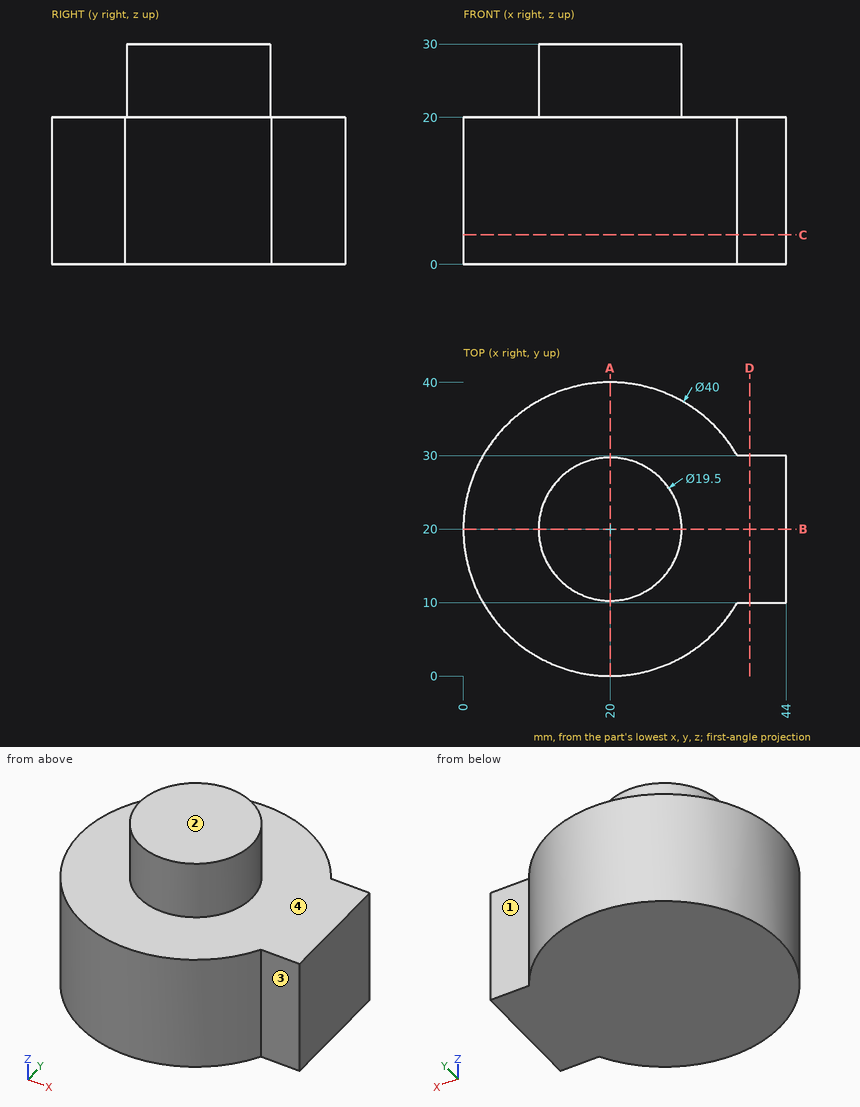
Check sheet for the drawn part. Datum: minimum x, y, z corner. Units: mm. A direction names the side the tool comes from. Coordinates: 2 decimals unless noted, no trailing zeros. Order: outer loops, then holes, each group sorted by start corner. A loop starts at its lowest first (then second) coordinate and runs counter-clockwise, first axis right, second up. Notation, with made-up numbers: M 40,30.5 L 88,30.5 A29 cw 88,55.5 Z; hole C -28.75,17 d8. An arc over 180 degrees is marked long. One line per question, with ' | ' between items. Start each with the question number.
Item 1: Cross-section at C-C on z = 4. Enter the section's corners in (x, y), then the cut area to 3 significant figures.
Item 2: Cross-section at D-D on x = 39. Enter the section's corners in (y, z), then the cut area to 3 significant figures.
Item 3: Cross-section at B-B on y = 20. Enter the section's corners in (x, z), then the cut area to 4 significant figures.
Item 4: Gauge pin test, flat ends, axial feed: pin 1 (10 mm diameter, centred on y = 6.5, z = 17, fed in from -X); pin 2 (4 mm diameter, centred on x = 26.5, y = 6, fed in from +Z); pin 3 (2 mm diameter, centred on x = 4.5, z = 17, fed in from +Y) (3 decimals). Record the tip position at first contact, or that the pin passes through.
Item 5: Material ranges on L1, parallel to X at y = 20.5, z = 27; L2, parallel to X at y = 20, z = 1.5; L3, parallel to Z at x = 32, y = 22.5, recorded low to high. Write a range as [from, to].
Item 6: Set-up check for the marked faces 1, 2, 3 and 4: record each of +Z, -Z, +X, -X, +Y, -Y from which the full face is reachable in a straight line by a thin tool's end or side.
Item 7: Cross-section at A-A on x = 20. Enter the section's corners in (y, z), then the cut area to 3 significant figures.
Findings:
1) outline: M 37.32,10 L 44,10 L 44,30 L 37.32,30 A20 ccw long Z | area: 1,350 mm²
2) outline: M 10,0 L 30,0 L 30,20 L 10,20 Z | area: 400 mm²
3) outline: M 0,0 L 44,0 L 44,20 L 29.75,20 L 29.75,30 L 10.25,30 L 10.25,20 L 0,20 Z | area: 1,075 mm²
4) pin 1: stops at x = 1.9 | pin 2: stops at z = 20 | pin 3: stops at y = 33.775
5) L1: x = [10.26, 29.74] | L2: x = [0, 44] | L3: z = [0, 20]
6) face 1: +Z, -Z, +X, +Y | face 2: +Z, +X, -X, +Y, -Y | face 3: +Z, -Z, +X, -Y | face 4: +Z
7) outline: M 0,0 L 40,0 L 40,20 L 29.75,20 L 29.75,30 L 10.25,30 L 10.25,20 L 0,20 Z | area: 995 mm²
